from build123d import *

# Parameters (mm, degrees)
SKETCH1_R                                         = 12.7
BOSS_EXTRUDE1_DEPTH                               = 12.7
SKETCH2_R                                         = 1.6256
CUT_EXTRUDE1_DEPTH                                = 9.525
BOSS_EXTRUDE6_START                               = -12.7
BOSS_EXTRUDE6_DEPTH                               = 12.7
SKETCH15_R                                        = 12.7
BOSS_EXTRUDE8_DEPTH                               = 12.7
SKETCH17_R                                        = 1.651
CUT_EXTRUDE4_DEPTH                                = 12.7
SKETCH18_R                                        = 3.81
CUT_EXTRUDE5_DEPTH                                = 10.9027722
SKETCH19_R                                        = 8.255
CUT_EXTRUDE6_DEPTH                                = 8.3627722
SKETCH20_R                                        = 9.525
CUT_EXTRUDE7_DEPTH                                = 5.1877722
SKETCH21_R                                        = 1.2192
CUT_EXTRUDE8_DEPTH                                = 4.3372278
SKETCH22_W                                        = 15.875
SKETCH22_H                                        = 25.4
CUT_EXTRUDE9_DEPTH                                = 33.534068682
SKETCH23_W                                        = 12.7
SKETCH23_H                                        = 25.4
BOSS_EXTRUDE9_DEPTH                               = 38.1
BOSS_EXTRUDE13_DEPTH                              = 12.7
FILLET1_R                                         = 12.7
CSK_FOR_8_FLAT_HEAD_MACHINE_SCREW_100_D           = 4.4958
CSK_FOR_8_FLAT_HEAD_MACHINE_SCREW_100_CSINK_D     = 8.4328
CSK_FOR_8_FLAT_HEAD_MACHINE_SCREW_100_CSINK_ANGLE = 100


with BuildPart() as part:
    # Sketch1 → Boss-Extrude1 (new body)
    with BuildSketch(Plane(origin=(0, 0, 0), x_dir=(1, 0, 0), z_dir=(0, 1, 0))):
        with Locations(Location((0, 0, 0), (0, 0, 270))):
            Circle(SKETCH1_R)
    extrude(amount=BOSS_EXTRUDE1_DEPTH)

    # Sketch2 → Cut-Extrude1 (cut)
    with BuildSketch(Plane.XZ):
        with Locations(Location((0, 0, 0), (0, 0, 270))):
            Circle(SKETCH2_R)
    extrude(amount=-CUT_EXTRUDE1_DEPTH, mode=Mode.SUBTRACT)

    # Sketch14 → Boss-Extrude6 (add)
    with BuildSketch(Plane(origin=(0, 12.7, 0), x_dir=(1, 0, 0), z_dir=(0, 1, 0)).offset(BOSS_EXTRUDE6_START)):
        with BuildLine():
            Line((15.875, 12.7), (0, 12.7))
            ThreePointArc((0, 12.7), (8.980256121, 8.980256121), (12.7, 0))
            ThreePointArc((12.7, 0), (8.980256121, -8.980256121), (0, -12.7))
            Line((0, -12.7), (15.875, -12.7))
            Line((15.875, -12.7), (15.875, 12.7))
        make_face()
    extrude(amount=BOSS_EXTRUDE6_DEPTH)

    # Sketch15 → Boss-Extrude8 (add)
    with BuildSketch(Plane(origin=(15.875, 0, 0), x_dir=(0, 0, -1), z_dir=(1, 0, 0))):
        with Locations((0, 25.4)):
            Circle(SKETCH15_R)
        with BuildLine():
            ThreePointArc((0, 12.7), (-8.980256121, 16.419743879), (-12.7, 25.4))
            Line((-12.7, 25.4), (-12.7, 12.7))
            Line((-12.7, 12.7), (0, 12.7))
        make_face()
        with BuildLine():
            Line((12.7, 12.7), (12.7, 25.4))
            ThreePointArc((12.7, 25.4), (8.980256121, 16.419743879), (0, 12.7))
            Line((0, 12.7), (12.7, 12.7))
        make_face()
    extrude(amount=-BOSS_EXTRUDE8_DEPTH)

    # Sketch17 → Cut-Extrude4 (cut)
    with BuildSketch(Plane.ZY.offset(-3.175)):
        with Locations((0, 25.4)):
            Circle(SKETCH17_R)
    extrude(amount=-CUT_EXTRUDE4_DEPTH, mode=Mode.SUBTRACT)

    # Sketch18 → Cut-Extrude5 (cut)
    with BuildSketch(Plane.ZY.offset(-3.175)):
        with Locations((0, 25.4)):
            Circle(SKETCH18_R)
    extrude(amount=-CUT_EXTRUDE5_DEPTH, mode=Mode.SUBTRACT)

    # Sketch19 → Cut-Extrude6 (cut)
    with BuildSketch(Plane.ZY.offset(-3.175)):
        with Locations((0, 25.4)):
            Circle(SKETCH19_R)
    extrude(amount=-CUT_EXTRUDE6_DEPTH, mode=Mode.SUBTRACT)

    # Sketch20 → Cut-Extrude7 (cut)
    with BuildSketch(Plane.ZY.offset(-3.175)):
        with Locations((0, 25.4)):
            Circle(SKETCH20_R)
    extrude(amount=-CUT_EXTRUDE7_DEPTH, mode=Mode.SUBTRACT)

    # Sketch21 → Cut-Extrude8 (cut)
    with BuildSketch(Plane.ZY.offset(-11.5377722)):
        with Locations((5.4599967, 25.4)):
            Circle(SKETCH21_R)
        with Locations((-5.4599967, 25.4)):
            Circle(SKETCH21_R)
    extrude(amount=-CUT_EXTRUDE8_DEPTH, mode=Mode.SUBTRACT)

    # Sketch22 → Cut-Extrude9 (cut, through all)
    with BuildSketch(Plane(origin=(0, 12.7, 0), x_dir=(1, 0, 0), z_dir=(0, 1, 0))):
        with Locations((-4.7625, 0)):
            Rectangle(SKETCH22_W, SKETCH22_H)
    extrude(amount=-CUT_EXTRUDE9_DEPTH, mode=Mode.SUBTRACT)

    # Sketch23 → Boss-Extrude9 (add)
    with BuildSketch(Plane.XZ):
        with Locations((9.525, 0)):
            Rectangle(SKETCH23_W, SKETCH23_H)
    extrude(amount=BOSS_EXTRUDE9_DEPTH)

    # Sketch28 → Boss-Extrude13 (add)
    with BuildSketch(Plane(origin=(15.875, 0, 0), x_dir=(0, 0, -1), z_dir=(1, 0, 0))):
        with BuildLine():
            ThreePointArc((-12.7, 25.4), (-12.276533056, 28.652189435), (-11.034372264, 31.687497812))
            Line((-11.034372264, 31.687497812), (-50.8, -38.1))
            Line((-50.8, -38.1), (-12.7, -38.1))
            Line((-12.7, -38.1), (-12.7, 25.4))
        make_face()
        with BuildLine():
            Line((50.8, -38.1), (11.034372264, 31.687497812))
            ThreePointArc((11.034372264, 31.687497812), (12.276533056, 28.652189435), (12.7, 25.4))
            Line((12.7, 25.4), (12.7, -38.1))
            Line((12.7, -38.1), (50.8, -38.1))
        make_face()
    extrude(amount=-BOSS_EXTRUDE13_DEPTH)

    # Fillet1
    fillet1_edges = [part.edges().sort_by_distance(p)[0] for p in [
        (9.525, -38.1, 50.8),
        (9.525, -38.1, -50.8),
    ]]
    fillet(fillet1_edges, radius=FILLET1_R)

    # CSK for #8 Flat Head Machine Screw (100)1 (through all)
    with Locations(Plane(origin=(15.875, 0, 0), x_dir=(0, 0, -1), z_dir=(1, 0, 0))):
        with Locations((28.946357905, -25.4), (-28.946357905, -25.4)):
            CounterSinkHole(CSK_FOR_8_FLAT_HEAD_MACHINE_SCREW_100_D / 2, CSK_FOR_8_FLAT_HEAD_MACHINE_SCREW_100_CSINK_D / 2, counter_sink_angle=CSK_FOR_8_FLAT_HEAD_MACHINE_SCREW_100_CSINK_ANGLE)


solid = part.part
The model under review builds one solid part; all positions refer to its coordinate system, in mm. A direction names the side the tool comes from. Coordinates: 2 decimals unless noted, no trailing zeros. Write each loop counter-clockwise with the first axis right and the second up, starting at its lowest first coordinate (ties: lowest second). Pieces come first, ordered by that corner, then holes. Notation, with made-up numbers: (23.25, 44) - (42.25, 44) arc R17 cw to (42.25, 68) - close; hole circle Ø6 at (80.5, 0). An arc over 180 degrees is marked (long way). Answer as a JSON object with one key per item and string values. Group by question number.
1. Clearance check with flat-ended pins moving along their axes: pin 1 Ø13 at (y, z) = (22.5, 2) entering from -X (3 decimals); pin 2 Ø11.5 at (y, z) = (25.4, 0) entering from -X; pin 3 Ø7 at (y, z) = (-25.4, 28.95) entering from +X; pin 4 Ø3 at (x, y) = (12.5, -8) entering from -Z. State where each tip first meets the part, or that it passes through.
2. Add section B-B (y = -25.4). Give the boundary of the cut face in (x, z) (3 decimals).
3. To check wall thickness, follow probe 1 along Z at (x, y) = (8.5, -25.4); probe 2 along Z at (x, y) = (13.5, 26); probe 3 along Y at (x, z) = (13.5, 0). State the ranges of each line that lie inside material, in increasing order.
4. Add section C-C (x = 9.5). Give the boundary of the cut face in (y, z) (1 decimal).
5. Add section A-A (z = 0). Give the boundary of the cut face in (x, y) (3 decimals).
6. Add section D-D (y = 25.4). Give the boundary of the cut face in (x, z) (3 decimals).
7. Mouldability with a two-part tool opening along Z and no side actions: class faces 1 (the face through (13.68, 25.77, -4.3)), 2 (the face through (9.6, 38.1, -0.2)), 3 (the face through (9.44, -31.62, 40.02)), 4 (the face through (10, -38.1, 0)) as pulls with the +Z half, pulls with the -Z half, needs draft (parallel to the pull), parting line crosses it, or undercut.
8. Machinability: for faces 5 (the face through (8.363, 34, 0)), 6 (the face through (3.175, -8, 1)), which of the approach directions +Z, -Z, +X, -X, +Y, -Y give a long, thin tool a straight path to every point of the face, cutting with its end or side? Answer none if there is none.
Findings:
{
 "1": {"pin 1": "x = 3.175", "pin 2": "x = 11.54", "pin 3": "x = 15.28", "pin 4": "z = -34.5"},
 "2": {"outline": "(3.175, -41.646) - (15.875, -41.646) - (15.875, -33.163) - (14.223, -31.194) - (3.175, -31.194) - close; (3.175, -26.698) - (14.223, -26.698) - (15.875, -24.73) - (15.875, 24.73) - (14.223, 26.698) - (3.175, 26.698) - close; (3.175, 31.194) - (14.223, 31.194) - (15.875, 33.163) - (15.875, 41.646) - (3.175, 41.646) - close"},
 "3": {"probe 1": "-41.65 to -31.19, -26.7 to 26.7, 31.19 to 41.65", "probe 2": "-14.28 to -6.52, -4.4 to -3.76, 3.76 to 4.4, 6.52 to 14.28", "probe 3": "-38.1 to 21.59, 29.21 to 38.1"},
 "4": {"outline": "(-38.1, -28.9) arc R12.7 ccw to (-19.1, -40) - (31.7, -11) arc R12.7 ccw to (31.7, 11) - (-19.1, 40) arc R12.7 ccw to (-38.1, 28.9) - close; hole circle Ø4.5 at (-25.4, -28.9); hole circle Ø4.5 at (-25.4, 28.9); hole circle Ø16.5 at (25.4, 0)"},
 "5": {"outline": "(3.175, -38.1) - (15.875, -38.1) - (15.875, 23.749) - (14.078, 23.749) - (14.078, 21.59) - (11.538, 21.59) - (11.538, 17.145) - (8.363, 17.145) - (8.363, 15.875) - (3.175, 15.875) - close; (3.175, 34.925) - (8.363, 34.925) - (8.363, 33.655) - (11.538, 33.655) - (11.538, 29.21) - (14.078, 29.21) - (14.078, 27.051) - (15.875, 27.051) - (15.875, 38.1) - (3.175, 38.1) - close"},
 "6": {"outline": "(3.175, -14.617) - (15.875, -14.617) - (15.875, -6.679) - (11.538, -6.679) - (11.538, -8.255) - (8.363, -8.255) - (8.363, -9.525) - (3.175, -9.525) - close; (3.175, 9.525) - (8.363, 9.525) - (8.363, 8.255) - (11.538, 8.255) - (11.538, 6.679) - (15.875, 6.679) - (15.875, 14.617) - (3.175, 14.617) - close; (11.538, -4.241) - (15.875, -4.241) - (15.875, -1.651) - (14.078, -1.651) - (14.078, -3.81) - (11.538, -3.81) - close; (11.538, 3.81) - (14.078, 3.81) - (14.078, 1.651) - (15.875, 1.651) - (15.875, 4.241) - (11.538, 4.241) - close"},
 "7": {"face 1": "undercut", "face 2": "parting line crosses it", "face 3": "pulls with the +Z half", "face 4": "needs draft"},
 "8": {"face 5": "-X", "face 6": "+Z, -Z, -X, +Y, -Y"}
}
